The model under review builds one solid part; all positions refer to its coordinate system, in mm. Face numbers are marked on the shaded views. A direction names the side the tool comes from. Coordinates: 2 decimals unless noted, no trailing zeros. Order: outer loops, then holes, each group sorted by start corner. A loop starts at its lowest first (then second) coordinate and runs counter-clockwise, first axis right, second up. Notation, with made-up numbers: (58, -2.5) -> (89, -2.5) arc R23 cw to (89, 32.5) -> close; hole circle Ø9 at (-35.5, -33.5). An arc over 180 degrees is marked (long way). Use CSV: the item, a comma, the result in double quotes. Start each with the question number.
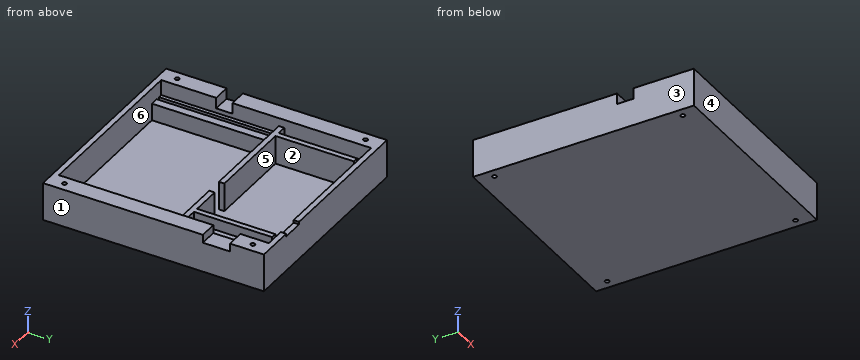
```python
from build123d import *

# Parameters (mm, degrees)
SKETCH1_W            = 81.5
SKETCH1_H            = 77
BOSS_EXTRUDE1_DEPTH  = 2
SKETCH2_W            = 81.5
SKETCH2_H            = 6.5
BOSS_EXTRUDE2_DEPTH  = 10
SKETCH3_W            = 22.3
SKETCH3_H            = 6.5
BOSS_EXTRUDE3_DEPTH  = 14
SKETCH4_W            = 53.2
SKETCH4_H            = 6.5
BOSS_EXTRUDE4_DEPTH  = 14
SKETCH5_W            = 81.5
SKETCH5_H            = 6.5
BOSS_EXTRUDE5_DEPTH  = 11
SKETCH6_W            = 59
SKETCH6_H            = 6.5
BOSS_EXTRUDE6_DEPTH  = 14
SKETCH7_W            = 12.5
SKETCH7_H            = 6.5
BOSS_EXTRUDE7_DEPTH  = 14
SKETCH8_W            = 2
SKETCH8_H            = 64
BOSS_EXTRUDE8_DEPTH  = 14
SKETCH9_W            = 2
SKETCH9_H            = 64
BOSS_EXTRUDE9_DEPTH  = 13
SKETCH10_W           = 2
SKETCH10_H           = 48.5
BOSS_EXTRUDE10_DEPTH = 14
SKETCH11_W           = 2
SKETCH11_H           = 7.5
BOSS_EXTRUDE11_DEPTH = 14
SKETCH12_W           = 77.5
SKETCH12_H           = 1.4
BOSS_EXTRUDE12_DEPTH = 8.3
SKETCH13_W           = 77.5
SKETCH13_H           = 3
BOSS_EXTRUDE13_DEPTH = 8.3
SKETCH14_W           = 77.5
SKETCH14_H           = 3
BOSS_EXTRUDE14_DEPTH = 8.3
SKETCH15_W           = 77.5
SKETCH15_H           = 1.5
BOSS_EXTRUDE15_DEPTH = 8.3
SKETCH16_W           = 2
SKETCH16_H           = 37.5
BOSS_EXTRUDE16_DEPTH = 12.5
SKETCH17_W           = 2
SKETCH17_H           = 16.5
BOSS_EXTRUDE17_DEPTH = 12.5
SKETCH18_W           = 28.9
SKETCH18_H           = 2
BOSS_EXTRUDE18_DEPTH = 12.5
SKETCH19_W           = 28.9
SKETCH19_H           = 2
BOSS_EXTRUDE19_DEPTH = 12.5
SKETCH20_R           = 0.8
CUT_EXTRUDE1_DEPTH   = 20
SKETCH21_R           = 0.8
CUT_EXTRUDE2_DEPTH   = 20
SKETCH22_R           = 0.8
CUT_EXTRUDE3_DEPTH   = 20
SKETCH23_R           = 0.8
CUT_EXTRUDE4_DEPTH   = 20


with BuildPart() as part:
    # Sketch1 → Boss-Extrude1 (new body)
    with BuildSketch(Plane(origin=(0, 0, 0), x_dir=(0, 1, 0), z_dir=(0, 0, 1))):
        with Locations((40.75, -38.5)):
            Rectangle(SKETCH1_W, SKETCH1_H)
    extrude(amount=BOSS_EXTRUDE1_DEPTH)

    # Sketch2 → Boss-Extrude2 (add)
    with BuildSketch(Plane(origin=(0, 0, 0), x_dir=(0, 1, 0), z_dir=(0, 0, 1))):
        with Locations((40.75, -3.25)):
            Rectangle(SKETCH2_W, SKETCH2_H)
    extrude(amount=BOSS_EXTRUDE2_DEPTH)

    # Sketch3 → Boss-Extrude3 (add)
    with BuildSketch(Plane(origin=(0, 0, 0), x_dir=(0, 1, 0), z_dir=(0, 0, 1))):
        with Locations((11.15, -3.25)):
            Rectangle(SKETCH3_W, SKETCH3_H)
    extrude(amount=BOSS_EXTRUDE3_DEPTH)

    # Sketch4 → Boss-Extrude4 (add)
    with BuildSketch(Plane(origin=(0, 0, 0), x_dir=(0, 1, 0), z_dir=(0, 0, 1))):
        with Locations((54.9, -3.25)):
            Rectangle(SKETCH4_W, SKETCH4_H)
    extrude(amount=BOSS_EXTRUDE4_DEPTH)

    # Sketch5 → Boss-Extrude5 (add)
    with BuildSketch(Plane(origin=(0, 0, 0), x_dir=(0, 1, 0), z_dir=(0, 0, 1))):
        with Locations((40.75, -73.75)):
            Rectangle(SKETCH5_W, SKETCH5_H)
    extrude(amount=BOSS_EXTRUDE5_DEPTH)

    # Sketch6 → Boss-Extrude6 (add)
    with BuildSketch(Plane(origin=(0, 0, 0), x_dir=(0, 1, 0), z_dir=(0, 0, 1))):
        with Locations((29.5, -73.75)):
            Rectangle(SKETCH6_W, SKETCH6_H)
    extrude(amount=BOSS_EXTRUDE6_DEPTH)

    # Sketch7 → Boss-Extrude7 (add)
    with BuildSketch(Plane(origin=(0, 0, 0), x_dir=(0, 1, 0), z_dir=(0, 0, 1))):
        with Locations((75.25, -73.75)):
            Rectangle(SKETCH7_W, SKETCH7_H)
    extrude(amount=BOSS_EXTRUDE7_DEPTH)

    # Sketch8 → Boss-Extrude8 (add)
    with BuildSketch(Plane(origin=(0, 0, 0), x_dir=(0, 1, 0), z_dir=(0, 0, 1))):
        with Locations((1, -38.5)):
            Rectangle(SKETCH8_W, SKETCH8_H)
    extrude(amount=BOSS_EXTRUDE8_DEPTH)

    # Sketch9 → Boss-Extrude9 (add)
    with BuildSketch(Plane(origin=(0, 0, 0), x_dir=(0, 1, 0), z_dir=(0, 0, 1))):
        with Locations((80.5, -38.5)):
            Rectangle(SKETCH9_W, SKETCH9_H)
    extrude(amount=BOSS_EXTRUDE9_DEPTH)

    # Sketch10 → Boss-Extrude10 (add)
    with BuildSketch(Plane(origin=(0, 0, 0), x_dir=(0, 1, 0), z_dir=(0, 0, 1))):
        with Locations((80.5, -30.75)):
            Rectangle(SKETCH10_W, SKETCH10_H)
    extrude(amount=BOSS_EXTRUDE10_DEPTH)

    # Sketch11 → Boss-Extrude11 (add)
    with BuildSketch(Plane(origin=(0, 0, 0), x_dir=(0, 1, 0), z_dir=(0, 0, 1))):
        with Locations((80.5, -66.75)):
            Rectangle(SKETCH11_W, SKETCH11_H)
    extrude(amount=BOSS_EXTRUDE11_DEPTH)

    # Sketch12 → Boss-Extrude12 (add)
    with BuildSketch(Plane(origin=(0, 0, 0), x_dir=(0, 1, 0), z_dir=(0, 0, 1))):
        with Locations((40.75, -7.2)):
            Rectangle(SKETCH12_W, SKETCH12_H)
    extrude(amount=BOSS_EXTRUDE12_DEPTH)

    # Sketch13 → Boss-Extrude13 (add)
    with BuildSketch(Plane(origin=(0, 0, 0), x_dir=(0, 1, 0), z_dir=(0, 0, 1))):
        with Locations((40.75, -10.8)):
            Rectangle(SKETCH13_W, SKETCH13_H)
    extrude(amount=BOSS_EXTRUDE13_DEPTH)

    # Sketch14 → Boss-Extrude14 (add)
    with BuildSketch(Plane(origin=(0, 0, 0), x_dir=(0, 1, 0), z_dir=(0, 0, 1))):
        with Locations((40.75, -66.1)):
            Rectangle(SKETCH14_W, SKETCH14_H)
    extrude(amount=BOSS_EXTRUDE14_DEPTH)

    # Sketch15 → Boss-Extrude15 (add)
    with BuildSketch(Plane(origin=(0, 0, 0), x_dir=(0, 1, 0), z_dir=(0, 0, 1))):
        with Locations((40.75, -69.75)):
            Rectangle(SKETCH15_W, SKETCH15_H)
    extrude(amount=BOSS_EXTRUDE15_DEPTH)

    # Sketch16 → Boss-Extrude16 (add)
    with BuildSketch(Plane(origin=(0, 0, 0), x_dir=(0, 1, 0), z_dir=(0, 0, 1))):
        with Locations((47.6, -27.25)):
            Rectangle(SKETCH16_W, SKETCH16_H)
    extrude(amount=BOSS_EXTRUDE16_DEPTH)

    # Sketch17 → Boss-Extrude17 (add)
    with BuildSketch(Plane(origin=(0, 0, 0), x_dir=(0, 1, 0), z_dir=(0, 0, 1))):
        with Locations((47.6, -60.25)):
            Rectangle(SKETCH17_W, SKETCH17_H)
    extrude(amount=BOSS_EXTRUDE17_DEPTH)

    # Sketch18 → Boss-Extrude18 (add)
    with BuildSketch(Plane(origin=(0, 0, 0), x_dir=(0, 1, 0), z_dir=(0, 0, 1))):
        with Locations((63.05, -13)):
            Rectangle(SKETCH18_W, SKETCH18_H)
    extrude(amount=BOSS_EXTRUDE18_DEPTH)

    # Sketch19 → Boss-Extrude19 (add)
    with BuildSketch(Plane(origin=(0, 0, 0), x_dir=(0, 1, 0), z_dir=(0, 0, 1))):
        with Locations((63.05, -64)):
            Rectangle(SKETCH19_W, SKETCH19_H)
    extrude(amount=BOSS_EXTRUDE19_DEPTH)

    # Sketch20 → Cut-Extrude1 (cut)
    with BuildSketch(Plane(origin=(0, 0, 0), x_dir=(0, 1, 0), z_dir=(0, 0, 1))):
        with Locations(Location((6, -3.25, 0), (0, 0, 270))):
            Circle(SKETCH20_R)
    extrude(amount=CUT_EXTRUDE1_DEPTH, mode=Mode.SUBTRACT)

    # Sketch21 → Cut-Extrude2 (cut)
    with BuildSketch(Plane(origin=(0, 0, 0), x_dir=(0, 1, 0), z_dir=(0, 0, 1))):
        with Locations(Location((75.5, -3.25, 0), (0, 0, 270))):
            Circle(SKETCH21_R)
    extrude(amount=CUT_EXTRUDE2_DEPTH, mode=Mode.SUBTRACT)

    # Sketch22 → Cut-Extrude3 (cut)
    with BuildSketch(Plane(origin=(0, 0, 0), x_dir=(0, 1, 0), z_dir=(0, 0, 1))):
        with Locations(Location((6, -73.75, 0), (0, 0, 270))):
            Circle(SKETCH22_R)
    extrude(amount=CUT_EXTRUDE3_DEPTH, mode=Mode.SUBTRACT)

    # Sketch23 → Cut-Extrude4 (cut)
    with BuildSketch(Plane(origin=(0, 0, 0), x_dir=(0, 1, 0), z_dir=(0, 0, 1))):
        with Locations(Location((75.5, -73.75, 0), (0, 0, 270))):
            Circle(SKETCH23_R)
    extrude(amount=CUT_EXTRUDE4_DEPTH, mode=Mode.SUBTRACT)


solid = part.part
```
Q1. Add section A-A, the plane y = 36. State the section outline as (x, z) points.
Q2. Add section D-D, the plane y = 52. State the section outline as (x, z) points.
Q3. To check wall thickness, follow probe 1 along X at (y, z) = (44.5, 8); probe 2 along Y at (x, z) = (44, 3.25); probe 3 along X at (y, z) = (6, 11). State the ranges of each line that lie inside material, in increasing order.
Q4. Draft analysis for pull direction Y (two halves, no side actions). For the marked faces 3, 4, 5 and 6, state which applies: +Y half, -Y half, draft (parallel to the pull), parting line (faces both ways), or undercut.
Q5. For the marked faces 1 and 2, list the 3-axis set-ups (+Z, -Z, +X, -X, +Y, -Y) from which the entire face can be reached by the end or side of a thin tool; tool diameter is ignored.
Q6. Add section C-C, the plane x = 17.5. State the section outline as (y, z) points, then the cut area to 3 significant figures.
Q7. Clearance check with flat-ended pins moving along their axes: pin 1 Ø6 at (x, z) = (35, 8) entering from -Y; pin 2 Ø2.5 at (x, y) = (10.5, 71) entering from +Z; pin 3 Ø1 at (x, y) = (57, 80.5) entering from +Z; pin 4 Ø2 at (x, y) = (44, 70.5) entering from +Z. State where each tip first meets the part, or that it passes through.
Q8. Add section B-B, the plane z = 6.5. State how many separate pieces and enclosed holes the cut face has, then the cut area to 3 significant figures.
Answer block:
1,outline,"(0, 0) -> (77, 0) -> (77, 14) -> (70.5, 14) -> (70.5, 8.3) -> (69, 8.3) -> (69, 2) -> (67.6, 2) -> (67.6, 8.3) -> (64.6, 8.3) -> (64.6, 2) -> (12.3, 2) -> (12.3, 8.3) -> (9.3, 8.3) -> (9.3, 2) -> (7.9, 2) -> (7.9, 8.3) -> (6.5, 8.3) -> (6.5, 14) -> (0, 14) -> close"
2,outline,"(0, 0) -> (77, 0) -> (77, 14) -> (70.5, 14) -> (70.5, 8.3) -> (69, 8.3) -> (69, 2) -> (67.6, 2) -> (67.6, 8.3) -> (65, 8.3) -> (65, 12.5) -> (63, 12.5) -> (63, 2) -> (14, 2) -> (14, 12.5) -> (12, 12.5) -> (12, 8.3) -> (9.3, 8.3) -> (9.3, 2) -> (7.9, 2) -> (7.9, 8.3) -> (6.5, 8.3) -> (6.5, 14) -> (0, 14) -> close"
3,probe 1,"x = 0 to 7.9, 9.3 to 12.3, 64.6 to 67.6, 69 to 77"
3,probe 2,"y = 0 to 2, 46.6 to 48.6, 79.5 to 81.5"
3,probe 3,"x = 0 to 2.45, 4.05 to 6.5, 70.5 to 72.95, 74.55 to 77"
4,face 3,"draft"
4,face 4,"-Y half"
4,face 5,"undercut"
4,face 6,"undercut"
5,face 1,"+Z, -Z, +X, +Y, -Y"
5,face 2,"+Z"
6,outline,"(0, 0) -> (81.5, 0) -> (81.5, 14) -> (79.5, 14) -> (79.5, 2) -> (48.6, 2) -> (48.6, 12.5) -> (46.6, 12.5) -> (46.6, 2) -> (2, 2) -> (2, 14) -> (0, 14) -> close"
6,area,"232 mm²"
7,pin 1,"stops at y = 0"
7,pin 2,"stops at z = 8.3"
7,pin 3,"stops at z = 13"
7,pin 4,"stops at z = 2"
8,separate pieces,"1"
8,enclosed holes,"7"
8,area,"2,190 mm²"
